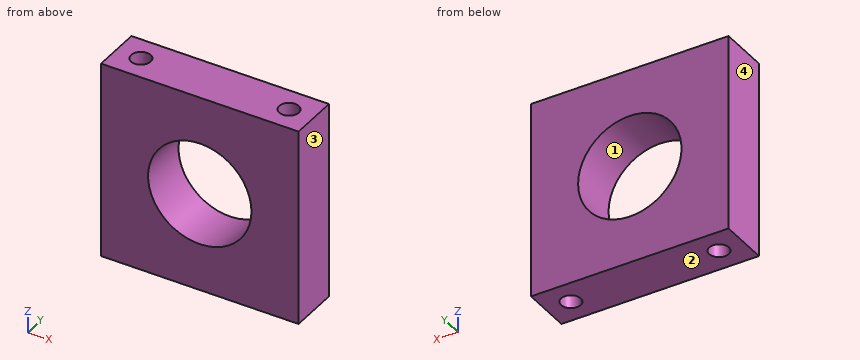
from build123d import *

# Parameters (mm, degrees)
F0_W     = 101.6
F0_H     = 101.6
F0_R     = 26.5811
F1_DEPTH = 25.4
F2_R     = 5.0419
F3_DEPTH = 101.601


with BuildPart() as f1:
    # F0 (on Front) → F1 (new body)
    with BuildSketch(Plane.XZ):
        Rectangle(F0_W, F0_H)
        Circle(F0_R, mode=Mode.SUBTRACT)
    extrude(amount=F1_DEPTH)

    # F2 (on face) → F3 (cut, through all)
    with BuildSketch(Plane(origin=(0, 0, -50.8), x_dir=(1, 0, 0), z_dir=(0, 0, -1))):
        with Locations((-38.1, 12.7)):
            Circle(F2_R)
        with Locations((38.1, 12.7)):
            Circle(F2_R)
    extrude(amount=-F3_DEPTH, mode=Mode.SUBTRACT)


solid = f1.part
Geometry: final body of the model. Coordinates: model frame, mm. Face numbers are marked on the shaded views. Round coordinates to 2 decimals unless told otherwise and drop trailing zeros. Order: outer loops, then holes, each group sorted by start corner. A loop starts at its lowest first (then second) coordinate and runs counter-clockwise, first axis right, second up. Notation, with made-up numbers: (60, 62.5) - (117, 62.5) arc R32 cw to (117, 94.5) - close; hole circle Ø11 at (38, -16.75). An arc over 180 degrees is marked (long way). Write each question's results on one line, items separated by ' | '.
Item 1: Material intervals for line 1 along X through (y, z) = (-12.7, -30); line 2 along Z through (x, y) = (0, -3); line 3 along X through (y, z) = (-11.5, -40), sorted ascending. Write a range as [from, to].
Completed:
line 1: [-50.8, -43.14], [-33.06, 33.06], [43.14, 50.8] | line 2: [-50.8, -26.58], [26.58, 50.8] | line 3: [-50.8, -43], [-33.2, 33.2], [43, 50.8]
Item 2: Section A-A, the plane z = 0. Return the cut outline in (x, y).
Completed:
outline: (-50.8, -25.4) - (-26.58, -25.4) - (-26.58, 0) - (-50.8, 0) - close; (26.58, -25.4) - (50.8, -25.4) - (50.8, 0) - (26.58, 0) - close; hole circle Ø10.08 at (-38.1, -12.7); hole circle Ø10.08 at (38.1, -12.7)
Item 3: Section C-C, the plane y = -12.7. Return the cut outline in (x, z).
Completed:
outline: (-50.8, -50.8) - (-43.14, -50.8) - (-43.14, 50.8) - (-50.8, 50.8) - close; (-33.06, -50.8) - (33.06, -50.8) - (33.06, 50.8) - (-33.06, 50.8) - close; (43.14, -50.8) - (50.8, -50.8) - (50.8, 50.8) - (43.14, 50.8) - close; hole circle Ø53.16 at (0, 0)
Item 4: Section B-B, the plane x = 38.1. Return the cut outline in (y, z).
Completed:
outline: (-25.4, -50.8) - (-17.74, -50.8) - (-17.74, 50.8) - (-25.4, 50.8) - close; (-7.66, -50.8) - (0, -50.8) - (0, 50.8) - (-7.66, 50.8) - close
Item 5: Mould query, pull axis X, two halves, no side actions, for the marked faces 1, 2, 3 and 4. Classes: pulls with the +X half, pulls with the -X half, needs draft (parallel to the pull), parting line crosses it, or undercut.
Completed:
face 1: undercut | face 2: needs draft | face 3: pulls with the +X half | face 4: pulls with the -X half
Item 6: Section D-D, the plane y = -5.5. Return the cut outline in (x, z), and give its area (3 significant figures).
Completed:
outline: (-50.8, -50.8) - (50.8, -50.8) - (50.8, 50.8) - (-50.8, 50.8) - close; hole circle Ø53.16 at (0, 0) | area: 8,100 mm^2
